```python
from build123d import *

# Parameters (mm, degrees)
BASPROSKE_W         = 10
BASPROSKE_H         = 11
TOOTHCUT_DEPTH      = 19.493242009
TEETHCUTS_COUNT     = 20
TEETHCUTS_ANGLE     = 342
BORSKE_R            = 0.4
BORE_DEPTH          = 50.0000508
SKETCH1_R           = 6.25
BOSS_EXTRUDE1_DEPTH = 5
FILLET1_R           = 0.5
CHAMFER1_SIZE       = 0.5
SKETCH4_R           = 2.5
CUT_EXTRUDE1_DEPTH  = 2.5


with BuildPart() as part:
    # BasProSke → Base-Revolve (revolve)
    with BuildSketch(Plane(origin=(0, 0, 0), x_dir=(1, 0, 0), z_dir=(0, 1, 0)), mode=Mode.PRIVATE) as base_revolve_sk:
        with Locations((5, 5.5)):
            Rectangle(BASPROSKE_W, BASPROSKE_H)
    revolve(base_revolve_sk.sketch.rotate(Axis((-10, 0, 0), (1, 0, 0)), 180), axis=Axis((-10, 0, 0), (1, 0, 0)))

    # TooCutSke → ToothCut (cut, through all)
    with BuildSketch(Plane(origin=(0, 0, 0), x_dir=(0, 0, -1), z_dir=(1, 0, 0))):
        with BuildLine():
            ThreePointArc((0.499924007, 8.734705318), (0, 8.749), (-0.499924007, 8.734705318))
            ThreePointArc((-0.499924007, 8.734705318), (-0.824302243, 9.905497836), (-1.485192705, 10.924909509))
            ThreePointArc((-1.485192705, 10.924909509), (0, 11.0254), (1.485192705, 10.924909509))
            ThreePointArc((1.485192705, 10.924909509), (0.824302243, 9.905497836), (0.499924007, 8.734705318))
        make_face()
    toothcut = extrude(amount=TOOTHCUT_DEPTH, mode=Mode.SUBTRACT)

    # TeethCuts: ToothCut ×20 about axis
    teethcuts_axis = Axis((-10, 0, 0), (1, 0, 0))
    for i in range(1, TEETHCUTS_COUNT):
        add(toothcut.rotate(teethcuts_axis, i * TEETHCUTS_ANGLE / (TEETHCUTS_COUNT - 1)), mode=Mode.SUBTRACT)

    # BorSke → Bore (cut, symmetric)
    with BuildSketch(Plane(origin=(0, 0, 0), x_dir=(0, 0, -1), z_dir=(1, 0, 0))):
        with Locations(Location((0, 0, 0), (0, 0, 180))):
            Circle(BORSKE_R)
    extrude(amount=BORE_DEPTH, both=True, mode=Mode.SUBTRACT)

    # Sketch1 → Boss-Extrude1 (add)
    with BuildSketch(Plane.ZY):
        with Locations(Location((0, 0, 0), (0, 0, 180))):
            Circle(SKETCH1_R)
    extrude(amount=BOSS_EXTRUDE1_DEPTH)

    # Fillet1
    fillet1_edges = [part.edges().sort_by_distance(p)[0] for p in [
        (0, 0, 6.25),
    ]]
    fillet(fillet1_edges, radius=FILLET1_R)

    # Chamfer1
    chamfer1_edges = [part.edges().sort_by_distance(p)[0] for p in [
        (-5, 0, 6.25),
    ]]
    chamfer(chamfer1_edges, length=CHAMFER1_SIZE)

    # Sketch4 → Cut-Extrude1 (cut)
    with BuildSketch(Plane.ZY.offset(5)):
        Circle(SKETCH4_R)
    extrude(amount=-CUT_EXTRUDE1_DEPTH, mode=Mode.SUBTRACT)


solid = part.part
```
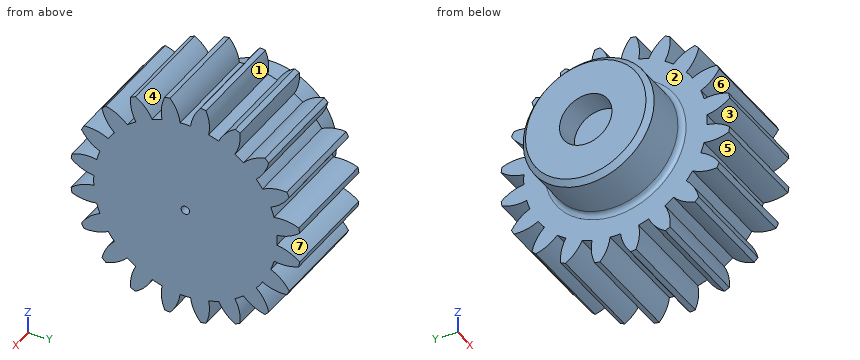
Build history of the part. All positions in model axes, mm. Face numbers are marked on the shaded views. A direction names the side the tool comes from. Coordinates: 2 decimals unless noted, no trailing zeros. Write each loop counter-clockwise with the first axis right and the second up, starting at its lowest first coordinate (ties: lowest second). Pieces come first, ordered by that corner, then holes.
1. Band-saw the part on D-D, the plane x = -3.25. Give the cut face in (y, z).
Answer block:
outline: circle Ø12.5 at (0, 0); hole circle Ø5 at (0, 0)
2. Drop flat-ended pins along their axis: pin 1 (1.5 mm diameter, centred on y = 1, z = 0.5, fed in from -X); pin 2 (8 mm diameter, centred on x = -2, y = -7.5, fed in from +Z); pin 3 (6 mm diameter, centred on x = 4.5, y = 6.5, fed in from -Z). Give the stop position or say it passes through.
Answer block:
pin 1: stops at x = -2.5
pin 2: stops at z = 9.92
pin 3: stops at z = -9.92
3. Pull direction Y, two halves, no side cores. Call the marked faces 1, 2 and 3: released by +Y, released by -Y, zero draft, split by the parting line, or undercut.
Answer block:
face 1: undercut
face 2: zero draft
face 3: released by -Y
4. 3-axis set-ups, long thin cutter, end or side, ignore diameter. For the marked faces 4, 5, 6 and 7: which of +Z, -Z, +X, -X, +Y, -Y reach the whole face in a straight line?
Answer block:
face 4: +Z, +X, -X
face 5: +X, -X
face 6: +X, -X, -Y
face 7: +X, -X, +Y
5. Band-saw the part on A-A, the plane y = 0. Give the cut face in (x, z), and give its area (3 significant figures).
Answer block:
outline: (-5, -5.75) - (-4.5, -6.25) - (-0.5, -6.25) arc R0.5 cw to (0, -6.75) - (0, -8.75) - (10, -8.75) - (10, -0.4) - (0, -0.4) - (0, 0.4) - (10, 0.4) - (10, 8.75) - (0, 8.75) - (0, 6.75) arc R0.5 cw to (-0.5, 6.25) - (-4.5, 6.25) - (-5, 5.75) - (-5, 2.5) - (-2.5, 2.5) - (-2.5, -2.5) - (-5, -2.5) - close
area: 217 mm2
6. Drill centre lines: probe 1 along Y at (x, z) = (5.25, -8.5); probe 2 along Y at (x, z) = (-4, 0); probe 3 along X at (y, z) = (-1.5, 9.5). Where is each one in solid material? Low to high.
Answer block:
probe 1: y = -5.16 to -3.36, -2.23 to 2.23, 3.36 to 5.16
probe 2: y = -6.25 to -2.5, 2.5 to 6.25
probe 3: x = 0 to 10
7. Band-saw the part on C-C, the plane y = 9.25. Give the cut face in (x, z), and give its area (3 significant figures).
Answer block:
outline: (0, -5.24) - (10, -5.24) - (10, -3.92) - (0, -3.92) - close; (0, -2.3) - (10, -2.3) - (10, -0.6) - (0, -0.6) - close; (0, 0.6) - (10, 0.6) - (10, 2.3) - (0, 2.3) - close; (0, 3.92) - (10, 3.92) - (10, 5.24) - (0, 5.24) - close
area: 60.4 mm2
